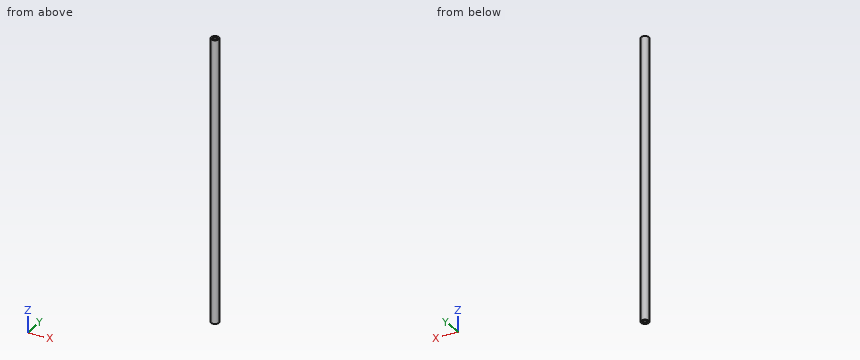
```python
from build123d import *

# Parameters (mm, degrees)
SKETCH_1_R          = 4
EXTRUDE_1_DEPTH     = 280
SKETCH_2_R          = 2
CUT_EXTRUDE_1_DEPTH = 10
CUT_EXTRUDE_START   = -10
SKETCH_3_R          = 2
CUT_EXTRUDE_2_DEPTH = 10


with BuildPart() as part:
    # 草图1 → 凸台-拉伸1 (new body)
    with BuildSketch(Plane.XY):
        Circle(SKETCH_1_R)
    extrude(amount=EXTRUDE_1_DEPTH)

    # 草图2 → 切除-拉伸1 (cut)
    with BuildSketch(Plane.XY.offset(280)):
        Circle(SKETCH_2_R)
    extrude(amount=-CUT_EXTRUDE_1_DEPTH, mode=Mode.SUBTRACT)

    # 草图3 → 切除-拉伸2 (cut)
    with BuildSketch(Plane(origin=(0, 0, 0), x_dir=(-1, 0, 0), z_dir=(0, 0, -1)).offset(CUT_EXTRUDE_START)):
        with Locations(Location((0, 0, 0), (0, 0, 180))):
            Circle(SKETCH_3_R)
    extrude(amount=CUT_EXTRUDE_2_DEPTH, mode=Mode.SUBTRACT)


solid = part.part
```
Check sheet for the modelled part. Datum: model origin and axes. Units: mm. Coordinates: 2 decimals unless noted, no trailing zeros. Write each loop counter-clockwise with the first axis right and the second up, starting at its lowest first coordinate (ties: lowest second). Pieces come first, ordered by that corner, then holes. Notation, with made-up numbers: (65, 3) -> (99, 3) arc R38 cw to (99, 41) -> close; hole circle Ø7 at (33.5, 58). An arc over 180 degrees is marked (long way). Use a Markdown table: item, result.
1. Sectioned sample at A-A (y = 0). Enter the section's corners in (x, z), plus the area to 3 significant figures.
Reported:
| item | result |
|---|---|
| outline | (-4, 0) -> (-2, 0) -> (-2, 10) -> (2, 10) -> (2, 0) -> (4, 0) -> (4, 280) -> (2, 280) -> (2, 270) -> (-2, 270) -> (-2, 280) -> (-4, 280) -> close |
| area | 2,160 mm2 |
2. Scan lines: line 1 along Y through (x, z) = (0, 6.5); line 2 along X through (y, z) = (0.5, 172.5); line 3 along Z through (x, y) = (1.5, -1). Record each from-to range of solid material in increasing order.
Reported:
| item | result |
|---|---|
| line 1 | y = -4 to -2, 2 to 4 |
| line 2 | x = -3.97 to 3.97 |
| line 3 | z = 10 to 270 |
3. Sectioned sample at B-B (x = -0.25). Enter the section's corners in (y, z).
Reported:
| item | result |
|---|---|
| outline | (-3.99, 0) -> (-1.98, 0) -> (-1.98, 10) -> (1.98, 10) -> (1.98, 0) -> (3.99, 0) -> (3.99, 280) -> (1.98, 280) -> (1.98, 270) -> (-1.98, 270) -> (-1.98, 280) -> (-3.99, 280) -> close |
4. Go/stop test with a flat-tipped pin: pin 1 Ø1.2 at (x, y) = (0, 0.5) entering from +Z. Record where the tip stops, or that it passes through.
Reported:
| item | result |
|---|---|
| pin 1 | stops at z = 270 |
5. Sectioned sample at C-C (z = 189.5). Enter the section's corners in (x, y), plus the area to 3 significant figures.
Reported:
| item | result |
|---|---|
| outline | circle Ø8 at (0, 0) |
| area | 50.3 mm2 |
